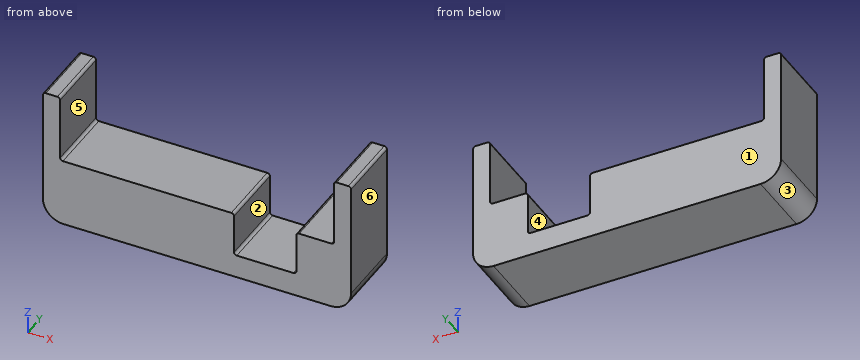
Autodesk Fusion 360 part; units mm, degrees
sketch "Sketch1" plane through (0, 0, 0) normal (0, 1, 0) x (1, 0, 0)
  line L0 (-22.5, 10) -> (22.5, 10)
  line L1 (22.5, 10) -> (22.5, -10)
  line L2 (22.5, -10) -> (-22.5, -10)
  line L3 (-22.5, -10) -> (-22.5, 10)
  line L4 (-22.5, 10) -> (22.5, -10) construction
  line L5 (22.5, 10) -> (-22.5, -10) construction
  dimension "d1" = 45
  dimension "d2" = 20
extrude "Extrude1" add sketch "Sketch1" along normal blind 10
sketch "Sketch2" plane through (0, 10, 0) normal (0, 1, 0) x (-1, 0, 0)
  line L0 (22.5, 10) -> (-22.5, 10)
  line L1 (-22.5, 10) -> (-22.5, -10)
  line L2 (-22.5, -10) -> (22.5, -10)
  line L3 (22.5, -10) -> (22.5, 10)
  line L4 (20, 10) -> (-20, 10)
  line L5 (-20, 10) -> (-20, 0)
  line L6 (-20, 0) -> (20, 0)
  line L7 (20, 0) -> (20, 10)
  dimension "d5" = 40
  dimension "d6" = 10
  dimension "d7" = 2.5
extrude "Extrude2" cut sketch "Sketch2" against normal through all contours L0 L4 L5 L6 L7
sketch "Sketch3" plane through (0, 10, 0) normal (0, 1, 0) x (-1, 0, 0)
  line L0 (20, 10) -> (20, 0)
  line L1 (20, 0) -> (-20, 0)
  line L2 (-20, 0) -> (-20, 10)
  line L3 (-20, 10) -> (-22.5, 10)
  line L4 (-22.5, 10) -> (-22.5, -10)
  line L5 (-22.5, -10) -> (22.5, -10)
  line L6 (22.5, -10) -> (22.5, 10)
  line L7 (22.5, 10) -> (20, 10)
  line L8 (-14.5, 0) -> (-5.4, 0)
  line L9 (-5.4, 0) -> (-5.4, -6.55)
  line L10 (-5.4, -6.55) -> (-14.5, -6.55)
  line L11 (-14.5, -6.55) -> (-14.5, 0)
  dimension "d9" = 9.1
  dimension "d12" = 6.55
  dimension "d13" = 5.5
extrude "Extrude3" cut sketch "Sketch3" against normal through all contours L1 L8 L9 L10 L11
fillet "Fillet1" radius 0.4 10 edges at (-20, 5, 10) (-20, 5, 0) (5.4, 5, 0) (5.4, 5, -6.55) (14.5, 5, -6.55) (14.5, 5, 0) (20, 5, 0) (20, 5, 10) (-22.5, 5, 10) (22.5, 5, 10)
fillet "Fillet2" radius 3 2 edges at (-22.5, 5, -10) (22.5, 5, -10)
Input: part model. Units: mm. Frame: model coordinates. Face numbers are marked on the shaded views. A direction names the side the tool comes from. Give positions to 0.01 mm unless a question says otherwise; leave off trailing zeros. Loops run counter-clockwise (first coordinate to the right, second up) from the corner with the lowest first, then second, coordinate; pieces in that order, holes last.
1) Mould query, pull axis X, two halves, no side actions, for the marked faces 1, 2, 3 and 4. Classes: released by +X, released by -X, zero draft, split by the parting line, or undercut.
A:
face 1: zero draft
face 2: undercut
face 3: released by -X
face 4: undercut
2) Section query A-A on z = 4. Return the cut outline in (x, y).
A:
outline: (-22.5, 0) - (-20, 0) - (-20, 10) - (-22.5, 10) - close; (20, 0) - (22.5, 0) - (22.5, 10) - (20, 10) - close
3) Section query B-B on y = 4. Return the cut outline in (x, z).
A:
outline: (-22.5, -7) arc R3 ccw to (-19.5, -10) - (19.5, -10) arc R3 ccw to (22.5, -7) - (22.5, 9.6) arc R0.4 ccw to (22.1, 10) - (20.4, 10) arc R0.4 ccw to (20, 9.6) - (20, 0.4) arc R0.4 cw to (19.6, 0) - (14.9, 0) arc R0.4 ccw to (14.5, -0.4) - (14.5, -6.15) arc R0.4 cw to (14.1, -6.55) - (5.8, -6.55) arc R0.4 cw to (5.4, -6.15) - (5.4, -0.4) arc R0.4 ccw to (5, 0) - (-19.6, 0) arc R0.4 cw to (-20, 0.4) - (-20, 9.6) arc R0.4 ccw to (-20.4, 10) - (-22.1, 10) arc R0.4 ccw to (-22.5, 9.6) - close
4) Line query: L1, parallel to X at y = 3.5, z = -4.25; L2, parallel to X at y = 5, z = 0.5; L3, parallel to X at y = 5.5, z = -7.25. Output: solid intervals per line, ascending.
A:
L1: x = -22.5 to 5.4, 14.5 to 22.5
L2: x = -22.5 to -20, 20 to 22.5
L3: x = -22.49 to 22.49
5) Section query D-D on x = 12. Return the cut outline in (y, z).
A:
outline: (0, -10) - (10, -10) - (10, -6.55) - (0, -6.55) - close
6) Contact query for a flat-ended pin moving along its axis: pin 1 (1.4 mm diameter, centred on x = 17, y = 7.5, fed in from +Z). Output: stop coordinate, or through.
A:
pin 1: stops at z = 0
7) Section query C-C on z = -1.5. Return the cut outline in (x, y), and give its area (3 significant figures).
A:
outline: (-22.5, 0) - (5.4, 0) - (5.4, 10) - (-22.5, 10) - close; (14.5, 0) - (22.5, 0) - (22.5, 10) - (14.5, 10) - close
area: 359 mm2
8) Reachability of the marked faces 5 and 6 from +Z, -Z, +X, -X, +Y, -Y: full face, straight path, thin tool, end or side. Return the list, or none.
A:
face 5: +Z, +Y, -Y
face 6: +Z, -Z, +X, +Y, -Y
